from build123d import *

# Parameters (mm, degrees)
F0_R     = 11
F0_R_2   = 9
F1_DEPTH = 7
F0_R_3   = 6
F0_R_4   = 4
F2_START = 1
F2_DEPTH = 5


with BuildPart() as f1:
    # F0 (on Top) → F1 (new body)
    with BuildSketch(Plane.XY):
        Circle(F0_R)
        Circle(F0_R_2, mode=Mode.SUBTRACT)
    extrude(amount=F1_DEPTH)



with BuildPart() as f1b:
    # F0 (on Top) → F1, piece 2 (new body)
    with BuildSketch(Plane.XY):
        Circle(F0_R_3)
        Circle(F0_R_4, mode=Mode.SUBTRACT)
    extrude(amount=F1_DEPTH)


with BuildPart() as f1_1:
    add(f1.part)

    add(f1b.part)  # F2 merges F1b
    # F0 (on Top) → F2 (join)
    with BuildSketch(Plane.XY.offset(F2_START)):
        Circle(F0_R_2)
        Circle(F0_R_3, mode=Mode.SUBTRACT)
    extrude(amount=F2_DEPTH)


solid = f1_1.part
Input: part model. Units: mm. Frame: model coordinates. A direction names the side the tool comes from. Coordinates: 2 decimals unless noted, no trailing zeros. Order: outer loops, then holes, each group sorted by start corner. A loop starts at its lowest first (then second) coordinate and runs counter-clockwise, first axis right, second up. Notation, with made-up numbers: M 44.25,70 L 76.25,70 A17 cw 76.25,77 Z; hole C 58,-26.5 d10. An arc over 180 degrees is marked long. Write item = value, one per line. Start each with the question number.
(1) Pull-direction query (Y, two-part tool) for faces 4 (the cylindrical face through (-2.38, -10.74, 3.45)), 5 (the flat face through (-1.42, -3.92, 0)), 6 (the flat face through (2, -6, 1)); classes: released by +Y, released by -Y, zero draft, split by the parting line, or undercut.
(2) Section C-C on z = 6.5. Output: boundary loops of the cut face in (x, y), and give its area (3 significant figures).
(3) Section D-D on z = 5. Output: boundary loops of the cut face in (x, y).
(4) Line query: line 1 along Y through (x, z) = (0, 0.7); line 2 along Y through (x, z) = (0, 4.5); line 3 along Y through (x, z) = (5.25, 6.75). Output: solid intervals per line, ascending. Write a range as [from, to].
(5) Section A-A on x = 0. Output: boundary loops of the cut face in (y, z).
(6) First-contact query: P1, Ø4, axis at x = -6, y = -3.5, coming from the -Z side; P2, Ø3, axis at x = -3.5, z = 2, coming from the +Y side. Flat tips, straight axial feed; report the tip coordinate or a pass-through.
(7) Reachability of faces 1 (the cylindrical face through (-5.994, 0.264, 0.493)), 2 (the flat face through (2, -9, 0)), 3 (the cylindrical face through (-1.172, 8.923, 6.493)) from +Z, -Z, +X, -X, +Y, -Y: full face, straight path, thin tool, end or side. Return the list, or none.
Result set:
q1.face_4 = split by the parting line
q1.face_5 = zero draft
q1.face_6 = undercut
q2.outline = C 0,0 d22; C 0,0 d12; hole C 0,0 d18; hole C 0,0 d8
q2.area = 188 mm²
q3.outline = C 0,0 d22; hole C 0,0 d8
q4.line_1 = [-11, -9], [-6, -4], [4, 6], [9, 11]
q4.line_2 = [-11, -4], [4, 11]
q4.line_3 = [-9.67, -7.31], [-2.9, 2.9], [7.31, 9.67]
q5.outline = M -11,0 L -9,0 L -9,1 L -6,1 L -6,0 L -4,0 L -4,7 L -6,7 L -6,6 L -9,6 L -9,7 L -11,7 Z; M 4,0 L 6,0 L 6,1 L 9,1 L 9,0 L 11,0 L 11,7 L 9,7 L 9,6 L 6,6 L 6,7 L 4,7 Z
q6.P1 = 0
q6.P2 = 10.82
q7.face_1 = -Z
q7.face_2 = -Z, +X, -X, +Y, -Y
q7.face_3 = +Z
